The listing builds one solid part. Answer for the finished solid, in the listing's coordinates (mm). A direction names the side the tool comes from. Round coordinates to 2 decimals unless told otherwise and drop trailing zeros. Write each loop counter-clockwise with the first axis right and the second up, starting at its lowest first coordinate (ties: lowest second). Pieces come first, ordered by that corner, then holes.
(1) A cutting plane is placed at D-D, the plane z = 33.5. Give the vertices of the cut face in (x, y).
(2) A cutting plane is placed at B-B, the plane y = 25. Give the vertices of the cut face in (x, z), and give its area (3 significant figures).
(3) A cutting plane is placed at A-A, the plane z = 14. Give the vertices of the cut face in (x, y).
(4) Each of these flat-tipped pins is pushed along its axis until it touches: pin 1 Ø2 at (y, z) = (23.5, 16) entering from -X; pin 2 Ø6 at (y, z) = (25, 25.5) entering from +X; pin 3 Ø1 at (y, z) = (9.5, 13.5) entering from +X. Where does it stop, or does it pass through?
(5) For faces 1 (the face through (11.282, 30, 28)), 2 (the face through (15, 40, 10)), determine the directions among +Z, -Z, +X, -X, +Y, -Y from which every point of the face is accessible in a straight line to the end or side of a thin tool.
(6) A cutting plane is placed at C-C, the plane x = 24.5. Give the vertices of the cut face in (y, z).
(7) The mould has two halves that part along X. Classify faces 3 (the face through (19.808, 30.14, 9.284)), 4 (the face through (28.718, 30, 28)), 5 (the face through (20, 0, 20)): +X half, -X half, draft (parallel to the pull), parting line (faces both ways), or undercut.
(8) Find the intervals of material crossed by probe 1 along Y at (x, z) = (22, 25.5); probe 2 along X at (y, z) = (24, 17); probe 3 along X at (y, z) = (27, 21), in increasing order.
from build123d import *

# Parameters (mm, degrees)
SKETCH1_W           = 40
SKETCH1_H           = 40
BOSS_EXTRUDE1_DEPTH = 40
CUT_EXTRUDE1_DEPTH  = 40
SKETCH3_W           = 2
SKETCH3_H           = 20
CUT_EXTRUDE2_DEPTH  = 40
CUT_EXTRUDE3_DEPTH  = 20


with BuildPart() as part:
    # Sketch1 → Boss-Extrude1 (new body)
    with BuildSketch(Plane.XY):
        with Locations((20, 20)):
            Rectangle(SKETCH1_W, SKETCH1_H)
    extrude(amount=BOSS_EXTRUDE1_DEPTH)

    # Sketch2 → Cut-Extrude1 (cut)
    with BuildSketch(Plane(origin=(0, 40, 0), x_dir=(1, 0, 0), z_dir=(0, 1, 0))):
        with BuildLine():
            Line((20, 0), (0, 0))
            Line((0, 0), (0, -20))
            ThreePointArc((0, -20), (5.857864376, -5.857864376), (20, 0))
        make_face()
        with BuildLine():
            Line((40, 0), (20, 0))
            ThreePointArc((20, 0), (34.142135624, -5.857864376), (40, -20))
            Line((40, -20), (40, 0))
        make_face()
        with BuildLine():
            Line((40, -40), (40, -20))
            ThreePointArc((40, -20), (34.142135624, -34.142135624), (20, -40))
            Line((20, -40), (40, -40))
        make_face()
        with BuildLine():
            ThreePointArc((20, -40), (5.857864376, -34.142135624), (0, -20))
            Line((0, -20), (0, -40))
            Line((0, -40), (20, -40))
        make_face()
    extrude(amount=-CUT_EXTRUDE1_DEPTH, mode=Mode.SUBTRACT)

    # Sketch3 → Cut-Extrude2 (cut)
    with BuildSketch(Plane(origin=(0, 0, 0), x_dir=(0, 0, -1), z_dir=(1, 0, 0))):
        with Locations((-39, 30)):
            Rectangle(SKETCH3_W, SKETCH3_H)
    extrude(amount=CUT_EXTRUDE2_DEPTH, mode=Mode.SUBTRACT)

    # Sketch4 → Cut-Extrude3 (cut)
    with BuildSketch(Plane(origin=(0, 40, 0), x_dir=(1, 0, 0), z_dir=(0, 1, 0))):
        with BuildLine():
            Line((11.282202113, -38), (11.282202113, -18))
            ThreePointArc((11.282202113, -18), (20, -9.282202113), (28.717797887, -18))
            Line((28.717797887, -18), (28.717797887, -38))
            Line((28.717797887, -38), (11.282202113, -38))
        make_face()
    extrude(amount=-CUT_EXTRUDE3_DEPTH, mode=Mode.SUBTRACT)


solid = part.part
Solutions:
1. outline: (5.24, 0) - (34.76, 0) - (34.76, 40) - (28.72, 40) - (28.72, 20) - (11.28, 20) - (11.28, 40) - (5.24, 40) - close
2. outline: (11.28, 18) - (11.28, 38) arc R20 ccw (long way) to (28.72, 38) - (28.72, 18) arc R8.72 cw to start
2. area: 765 mm2
3. outline: (0.92, 0) - (39.08, 0) - (39.08, 40) - (27.75, 40) - (27.75, 20) - (12.25, 20) - (12.25, 40) - (0.92, 40) - close
4. pin 1: stops at x = 0.23
4. pin 2: stops at x = 39.84
4. pin 3: stops at x = 39.08
5. face 1: +Z, +Y
5. face 2: +Z, -Z, +X, -X, +Y
6. outline: (0, 0.51) - (40, 0.51) - (40, 10.53) - (20, 10.53) - (20, 39.49) - (0, 39.49) - close
7. face 3: undercut
7. face 4: undercut
7. face 5: draft
8. probe 1: y = 0 to 20
8. probe 2: x = 0.23 to 11.34, 28.66 to 39.77
8. probe 3: x = 0.03 to 11.28, 28.72 to 39.97
